```python
from build123d import *

# Parameters (mm, degrees)
F0_W     = 84
F0_H     = 30
F1_DEPTH = 250
F2_W     = 80
F2_H     = 50.6085516345
F3_DEPTH = 250.001
F4_R     = 5
F5_DEPTH = 5
F6_W     = 76
F6_H     = 1.5
F7_DEPTH = 25.4
F8_F1_R  = 29.9999


# Not quite as in the source:
# - a fillet or chamfer is up to 0.001 mm smaller than in the source, because OpenCascade refuses the exact size


with BuildPart() as f1:
    # F0 (on Front) → F1 (new body)
    with BuildSketch(Plane.XZ):
        with Locations((-42, 15)):
            Rectangle(F0_W, F0_H)
    extrude(amount=-F1_DEPTH)

    # F2 (on Front) → F3 (cut, through all)
    with BuildSketch(Plane.XZ):
        with Locations((-42, 30.3042758173)):
            Rectangle(F2_W, F2_H)
    extrude(amount=-F3_DEPTH, mode=Mode.SUBTRACT)

    # F4 (on face) → F5 (join)
    with BuildSketch(Plane(origin=(0, 0, 0), x_dir=(1, 0, 0), z_dir=(0, 0, -1))):
        with Locations((-75.0694796443, -9.1842794791)):
            Circle(F4_R)
        with Locations((-9.0694796443, -9.1842794791)):
            Circle(F4_R)
        with BuildLine():
            add(Edge.make_bspline(
                [(-42, -228.9691147673), (-42, -236.5294238205), (-42, -242.7407619737), (-42, -247.3817589414)],
                knots=[0.7062379003, 0.7062379003, 0.7062379003, 0.7062379003, 0.8221337183, 0.8221337183, 0.8221337183, 0.8221337183], degree=3))
            add(Edge.make_bspline(
                [(-42, -228.9691147673), (-72.1999239177, -228.6668722572), (-72.1999239177, -238.1754368544), (-72.1999239177, -247.6840014516), (-42, -247.3817589414)],
                knots=[1.5390046272, 1.5390046272, 1.5390046272, 3.1415926536, 3.1415926536, 4.74418068, 4.74418068, 4.74418068], degree=2, weights=[1, 0.695777858, 1, 0.695777858, 1]))
        make_face()
        with BuildLine():
            add(Edge.make_bspline(
                [(-42, -247.3817589414), (-13.660820201, -247.0981388613), (-13.660820201, -238.1754368544)],
                knots=[4.74418068, 4.74418068, 4.74418068, 6.2831853072, 6.2831853072, 6.2831853072], degree=2, weights=[1, 0.7182570377, 1]))
            add(Edge.make_bspline(
                [(-13.660820201, -238.1754368544), (-13.660820201, -229.2527348474), (-42, -228.9691147673)],
                knots=[0, 0, 0, 1.5390046272, 1.5390046272, 1.5390046272], degree=2, weights=[1, 0.7182570377, 1]))
            add(Edge.make_bspline(
                [(-42, -228.9691147673), (-42, -236.5294238205), (-42, -242.7407619737), (-42, -247.3817589414)],
                knots=[0.7062379003, 0.7062379003, 0.7062379003, 0.7062379003, 0.8221337183, 0.8221337183, 0.8221337183, 0.8221337183], degree=3))
        make_face()
    extrude(amount=F5_DEPTH)

    # F6 (on face) → F7 (cut)
    with BuildSketch(Plane.XY.offset(5)):
        with Locations((-42, 213.1024897098)):
            Rectangle(F6_W, F6_H)
        with Locations((-42.0274770269, 185.1625032207)):
            Rectangle(F6_W, F6_H)
        with Locations((-42.0549540537, 157.2225167316)):
            Rectangle(F6_W, F6_H)
        with Locations((-42.1648621612, 45.462570775)):
            Rectangle(F6_W, F6_H)
        with Locations((-42.1373851343, 73.4025572642)):
            Rectangle(F6_W, F6_H)
        with Locations((-42.1099081074, 101.3425437533)):
            Rectangle(F6_W, F6_H)
        with Locations((-42.0824310806, 129.2825302424)):
            Rectangle(F6_W, F6_H)
    extrude(amount=-F7_DEPTH, mode=Mode.SUBTRACT)

    # F8: fillet of radius 30 on 2 edges, made by hand

    # F8_f1 (radius 30 in the source; OpenCascade refuses exactly that, so slightly less here)
    f8_f1_edges = [f1.edges().sort_by_distance(p)[0] for p in [
        (-83, 0, 30),
    ]]
    fillet(f8_f1_edges, radius=F8_F1_R)


solid = f1.part
```
Design review of the part built by this model. Coordinates are the model's own, in mm. A direction names the side the tool comes from. Give positions to 0.01 mm unless a question says otherwise; leave off trailing zeros. Order: outer loops, then holes, each group sorted by start corner. A loop starts at its lowest first (then second) coordinate and runs counter-clockwise, first axis right, second up. Notation, with made-up numbers: (24, 88.25) -> (71, 88.25) arc R13 cw to (71, 111.25) -> close; hole circle Ø7 at (48.25, 14.5). An arc over 180 degrees is marked (long way). Write each question's results on one line, items separated by ' | '. Start each with the question number.
Q1. Wall thickness on L1, parallel to X at y = 104.5, z = 22.5; L2, parallel to Z at x = -60, y = 28.5; L3, parallel to Y at x = -40, z = -1: over which ranges is each line inside the solid? List them lowest first. Write a range as from..to.
Q2. Add section B-B on y = 83. Give the boundary of the cut face in (x, z).
Q3. For pin 1 (6 mm diameter, centred on x = -31, y = 218.5, fed in from -Z); pin 2 (4 mm diameter, centred on x = -48, z = 3.5, fed in from -Y), all flat-tipped, find the tip position at first contact; note any pin that passes through.
Q4. Add section A-A on z = 23.5. Give the boundary of the cut face in (x, y).
Q5. Mouldability with a two-part tool opening along X and no side actions: class faces 1 (the flat face through (0, 123, 15)), 2 (the cylindrical face through (-14.065, 8.964, -2.465)), 3 (the flat face through (-43, 238, -5)) as +X half, -X half, draft (parallel to the pull), parting line (faces both ways), or undercut.
Q6. Machinability: for faces 4 (the cylindrical face through (-41.804, 0.333, 4.457)), 5 (the cylindrical face through (-80.065, 8.964, -2.465)), 6 (the flat face through (-2, 123, 17)), 7 (the flat face through (-43, 74.153, 3)), which of the approach directions +Z, -Z, +X, -X, +Y, -Y give a long, thin tool a straight path to every point of the face, cutting with its end or side? Answer none if there is none.
Q7. Add section C-C on x = -61.5. State how many separate pieces and enclosed holes the cut face has, and give its area (3 significant figures).
Found:
1) L1: x = -84..-82, -2..0 | L2: z = 0..5 | L3: y = 229.01..247.34
2) outline: (-84, 0) -> (0, 0) -> (0, 30) -> (-2, 30) -> (-2, 5) -> (-82, 5) -> (-82, 30) -> (-84, 30) -> close
3) pin 1: stops at z = 0 | pin 2: stops at y = 0.04
4) outline: (-84, 11.35) -> (-82, 11.35) -> (-82, 250) -> (-84, 250) -> close; (-2, 11.35) -> (0, 11.35) -> (0, 250) -> (-2, 250) -> close
5) face 1: +X half | face 2: undercut | face 3: draft
6) face 4: +Z, +X, -X, -Y | face 5: -Z | face 6: +Z, +Y, -Y | face 7: +Z, -Z
7) separate pieces: 8 | enclosed holes: 0 | area: 1,270 mm2
